Geometry: final body of the model. Coordinates: model frame, mm. A direction names the side the tool comes from. Round coordinates to 2 decimals unless told otherwise and drop trailing zeros. Loops run counter-clockwise (first coordinate to the right, second up) from the corner with the lowest first, then second, coordinate; pieces in that order, holes last. Notation, with made-up numbers: M 68,36.5 L 90,36.5 A17 ccw 90,57.5 Z; hole C 45.5,11 d1. An arc over 180 degrees is marked long. Return JSON: item names as keys, results as strings.
from build123d import *

# Parameters (mm, degrees)
SKETCH2_W               = 25
SKETCH2_H               = 8
SKETCH2_3_W             = 25
SKETCH2_3_H             = 8
BOSS_EXTRUDE1_DEPTH     = 17
FILLET2_R               = 5
SKETCH3_R               = 6.5
CUT_EXTRUDE2_DEPTH      = 4
CUT_EXTRUDE2_DEPTH_BACK = 1
SKETCH4_R               = 15
SKETCH4_R_2             = 6.5
BOSS_EXTRUDE2_DEPTH     = 5
SKETCH5_R               = 2.05
CUT_EXTRUDE3_DEPTH      = 3


with BuildPart() as part:
    # Sketch1 for Loft1 → Loft1 section 0
    with BuildSketch(Plane(origin=(0, 0, 0), x_dir=(0, 0, -1), z_dir=(1, 0, 0))):
        with BuildLine():
            # circular arc as an exact rational Bezier (weights 1, cos(half-angle), 1)
            Bezier((-14.286362208, -4.571635907), (0, -49.216517801), (14.286362208, -4.571635907), weights=[1, 0.304775727, 1])
            Bezier((14.286362208, -4.571635907), (15.749285698, 0), (14.286362208, 4.571635907), weights=[1, 0.952424147, 1])
            Bezier((14.286362208, 4.571635907), (0, 49.216517801), (-14.286362208, 4.571635907), weights=[1, 0.304775727, 1])
            Bezier((-14.286362208, 4.571635907), (-15.749285698, 0), (-14.286362208, -4.571635907), weights=[1, 0.952424147, 1])
        make_face()
    # Sketch2 → Loft1 section 1
    with BuildSketch(Plane(origin=(8.5, 0, 0), x_dir=(0, 0, -1), z_dir=(1, 0, 0))):
        Rectangle(SKETCH2_W, SKETCH2_H)
    loft()

    # Sketch2_3 → Boss-Extrude1 (add)
    with BuildSketch(Plane(origin=(8.5, 0, 0), x_dir=(0, 0, -1), z_dir=(1, 0, 0))):
        Rectangle(SKETCH2_3_W, SKETCH2_3_H)
    extrude(amount=BOSS_EXTRUDE1_DEPTH)

    # Fillet2
    fillet2_edges = [part.edges().sort_by_distance(p)[0] for p in [
        (25.5, 0, 12.5),
        (25.5, 0, -12.5),
    ]]
    fillet(fillet2_edges, radius=FILLET2_R)

    # Sketch3 → Cut-Extrude2 (cut, two sides)
    with BuildSketch(Plane(origin=(0, 0, 0), x_dir=(1, 0, 0), z_dir=(0, 1, 0))) as cut_extrude2_sk:
        with Locations(Location((15, 0, 0), (0, 0, 180))):
            Circle(SKETCH3_R)
    extrude(amount=CUT_EXTRUDE2_DEPTH, mode=Mode.SUBTRACT)
    extrude(cut_extrude2_sk.sketch, amount=-CUT_EXTRUDE2_DEPTH_BACK, mode=Mode.SUBTRACT)

    # Sketch4 → Boss-Extrude2 (add)
    with BuildSketch(Plane.ZY):
        with Locations(Location((0, 0, 0), (0, 0, 162.255321529))):
            Circle(SKETCH4_R)
        Circle(SKETCH4_R_2, mode=Mode.SUBTRACT)
    extrude(amount=BOSS_EXTRUDE2_DEPTH)

    # Sketch5 → Cut-Extrude3 (cut)
    with BuildSketch(Plane(origin=(0, -1, 0), x_dir=(1, 0, 0), z_dir=(0, 1, 0))):
        with Locations(Location((15, 0, 0), (0, 0, 270))):
            Circle(SKETCH5_R)
    extrude(amount=-CUT_EXTRUDE3_DEPTH, mode=Mode.SUBTRACT)


solid = part.part
Q1. Reachability of faces 1 (the flat face through (19, -4, 0)), 2 (the flat face through (14, 0, 12.5)), 3 (the flat face through (0, 0, 0)), 4 (the flat face through (17, -1, 2)) from +Z, -Z, +X, -X, +Y, -Y: full face, straight path, thin tool, end or side. Return the list, or none.
Determined:
{"face 1": "+Z, -Z, +X, -Y", "face 2": "+Z, +X, +Y, -Y", "face 3": "-X", "face 4": "+Y"}
Q2. Pull-direction query (Y, two-part tool) for faces 5 (the cylindrical face through (-2.465, -3.955, -5.158)), 6 (the cylindrical face through (12.999, -2.479, -0.444)), 7 (the flat face through (23, 4, 0)); classes: pulls with the +Y half, pulls with the -Y half, needs draft (parallel to the pull), parting line crosses it, or undercut.
Determined:
{"face 5": "undercut", "face 6": "needs draft", "face 7": "pulls with the +Y half"}
Q3. Material intervals for L1, parallel to Y at x = -3.95, z = 0; L2, parallel to Z at x = 15, y = 2.2; L3, parallel to X at y = -3, z = 0, sorted ascending.
Determined:
{"L1": "y = -15 to -6.5, 6.5 to 15", "L2": "z = -12.5 to -6.5, 6.5 to 12.5", "L3": "x = 0 to 12.95, 17.05 to 25.5"}
Q4. Pin query (flat end, axial travel): pin 1 (8 mm diameter, centred on x = 10, z = 1, fed in from -Y); pin 2 (12 mm diameter, centred on x = 21.5, y = -4, fed in from +Z); pin 3 (8 mm diameter, centred on x = 22.5, z = 6, fed in from -Y); pin 4 (2.5 mm diameter, centred on x = 15, z = 0, fed in from +Y). Return the tip coordinate at first contact, or that it passes through.
Determined:
{"pin 1": "stops at y = -7.22", "pin 2": "stops at z = 12.5", "pin 3": "stops at y = -4", "pin 4": "passes through"}
Q5. Section query B-B (x = 24.5). Output: boundary loops of the cut face in (y, z).
Determined:
{"outline": "M -4,-10.5 L 4,-10.5 L 4,10.5 L -4,10.5 Z"}
Q6. Section query A-A (x = 15). Output: boundary loops of the cut face in (y, z).
Determined:
{"outline": "M -4,-12.5 L 4,-12.5 L 4,-6.5 L -1,-6.5 L -1,-2.05 L -4,-2.05 Z; M -4,2.05 L -1,2.05 L -1,6.5 L 4,6.5 L 4,12.5 L -4,12.5 Z"}
